```python
from build123d import *

# Parameters (mm, degrees)
F3_DEPTH      = 5.97
F3_DEPTH_BACK = 5.97
F4_R          = 1.778
F5_DEPTH      = 5.97
F5_DEPTH_BACK = 5.97


with BuildPart() as f1:
    # F0 (on Front) → F1 (revolve)
    with BuildSketch(Plane.XZ):
        with BuildLine():
            Line((0, 26.543), (0, 0))
            Line((0, 0), (4.3815, 0))
            Line((4.3815, 0), (4.3815, 18.161))
            Line((4.3815, 18.161), (4.8895, 18.161))
            Line((4.8895, 18.161), (4.8895, 19.685))
            Line((4.8895, 19.685), (5.969, 19.685))
            Line((5.969, 19.685), (5.969, 20.828))
            Line((5.969, 20.828), (5.969, 22.098))
            Line((5.969, 22.098), (3.4925, 22.098))
            Line((3.4925, 22.098), (3.4925, 26.543))
            Line((3.4925, 26.543), (2.921, 26.543))
            Line((2.921, 26.543), (2.921, 29.083))
            ThreePointArc((2.921, 29.083), (2.9930503377, 32.5522788465), (0, 34.3080512242))
            Line((0, 34.3080512242), (0, 26.543))
        make_face()
    revolve(axis=Axis((0, 0, 28.8581177592), (0, 0, -1)))

    # F2 (on Right) → F3 (cut, two sides)
    with BuildSketch(Plane.YZ) as f3_sk:
        Polygon((-3.4925, 26.543), (-1.7145, 26.543), (-1.7145, 36.703), (-6.1595, 36.703), (-6.1595, 26.543), align=None)
        Polygon((3.4925, 26.543), (6.1595, 26.543), (6.1595, 36.703), (1.7145, 36.703), (1.7145, 26.543), align=None)
    extrude(amount=F3_DEPTH, mode=Mode.SUBTRACT)
    extrude(f3_sk.sketch, amount=-F3_DEPTH_BACK, mode=Mode.SUBTRACT)

    # F4 (on Front) → F5 (cut, two sides)
    with BuildSketch(Plane.XZ) as f5_sk:
        with Locations((0, 30.8790512242)):
            Circle(F4_R)
    extrude(amount=-F5_DEPTH, mode=Mode.SUBTRACT)
    extrude(f5_sk.sketch, amount=F5_DEPTH_BACK, mode=Mode.SUBTRACT)


solid = f1.part
```
Read the model definition and answer for the solid it produces. Units are mm, in the model's axes. A direction names the side the tool comes from. Round coordinates to 2 decimals unless told otherwise and drop trailing zeros. Write each loop counter-clockwise with the first axis right and the second up, starting at its lowest first coordinate (ties: lowest second). Pieces come first, ordered by that corner, then holes. Notation, with made-up numbers: (13, 35.5) - (31, 35.5) arc R34 ccw to (31, 72.5) - close; hole circle Ø3 at (76.5, 5). An arc over 180 degrees is marked (long way). Use CSV: the item, a comma, the result in double quotes.
Q1. Find section B-B, the plane y = 0.5. Write down the section's boundary in (x, z) (3 decimals).
Values:
outline,"(-5.948, 19.685) - (-4.864, 19.685) - (-4.864, 18.161) - (-4.353, 18.161) - (-4.353, 0) - (4.353, 0) - (4.353, 18.161) - (4.864, 18.161) - (4.864, 19.685) - (5.948, 19.685) - (5.948, 22.098) - (3.457, 22.098) - (3.457, 26.543) - (2.878, 26.543) - (2.878, 29.083) arc R3.392 ccw (long way) to (-2.878, 29.083) - (-2.878, 26.543) - (-3.457, 26.543) - (-3.457, 22.098) - (-5.948, 22.098) - close; hole circle Ø3.556 at (0, 30.879)"
Q2. Find section D-D, the plane y = -2.75. Write down the section's boundary in (x, z) (3 decimals), then the cut area to 3 significant figures.
Values:
outline,"(-5.298, 19.685) - (-4.043, 19.685) - (-4.043, 18.161) - (-3.411, 18.161) - (-3.411, 0) - (3.411, 0) - (3.411, 18.161) - (4.043, 18.161) - (4.043, 19.685) - (5.298, 19.685) - (5.298, 22.098) - (2.153, 22.098) - (2.153, 26.543) - (-2.153, 26.543) - (-2.153, 22.098) - (-5.298, 22.098) - close"
area,"181 mm²"
Q3. Determine the mould class of faces 1 (the cylindrical face through (-0.455, -3.463, 24.352)), 2 (the cylindrical face through (2.92, 0.03, 27.83)), 3 (the flat face through (0, 2, 26.543)), 4 (the cylindrical face through (-0.231, -0.024, 32.642)) for opening direction X: +X half, -X half, draft (parallel to the pull), parting line (faces both ways), or undercut.
Values:
face 1,"parting line"
face 2,"+X half"
face 3,"draft"
face 4,"undercut"
Q4. Each of these flat-tipped pins is pushed along its axis until it touches: pin 1 Ø4 at (x, z) = (0, 30.88) entering from +Y; pin 2 Ø1 at (x, z) = (-1, 24) entering from -Y; pin 3 Ø6 at (x, z) = (3, 7.5) entering from +Y; pin 4 Ø6 at (x, y) = (2, -2) entering from +Z. Where does it stop, or does it pass through?
Values:
pin 1,"stops at y = 1.71"
pin 2,"stops at y = -3.46"
pin 3,"stops at y = 4.38"
pin 4,"stops at z = 34.31"
Q5. A tool of negligible diameter and unlimited length cuts with its end or side. For faces 5 (the flat face through (3, 3, 22.098)), 6 (the cylindrical face through (-1.06, 4.773, 18.934)), 7 (the flat face through (0, -1.714, 28.5)), from which of +Z, -Z, +X, -X, +Y, -Y can it reach the whole face along a straight path? Write none if from no direction.
Values:
face 5,"+Z"
face 6,"-Z"
face 7,"+Z, +X, -X, -Y"
Q6. Straight lines are drawn through the part: line 1 along Z through (x, y) = (5.5, -1.75) (3 decimals); line 2 along Z through (x, y) = (0, -1); line 3 along Y through (x, z) = (0, 14). For each, find the intervals that lie inside material, in ascending order.
Values:
line 1,"z = 19.685 to 22.098"
line 2,"z = 0 to 29.1, 32.66 to 34.16"
line 3,"y = -4.38 to 4.38"
Q7. Find section C-C, the plane z = 18.5. Write down the section's boundary in (x, y).
Values:
outline,"circle Ø9.78 at (0, 0)"
Q8. Find section A-A, the plane x = 0. Write down the section's boundary in (y, z) (1 decimal).
Values:
outline,"(-6, 19.7) - (-4.9, 19.7) - (-4.9, 18.2) - (-4.4, 18.2) - (-4.4, 0) - (4.4, 0) - (4.4, 18.2) - (4.9, 18.2) - (4.9, 19.7) - (6, 19.7) - (6, 22.1) - (3.5, 22.1) - (3.5, 26.5) - (1.7, 26.5) - (1.7, 29.1) - (-1.7, 29.1) - (-1.7, 26.5) - (-3.5, 26.5) - (-3.5, 22.1) - (-6, 22.1) - close; (-1.7, 32.7) - (1.7, 32.7) - (1.7, 33.8) arc R3.4 ccw to (-1.7, 33.8) - close"
